Geometry: see drawing. Coordinates: mm, zero at the bounding-box minimum. A direction names the side the tool comes from. Round coordinates to 2 decimals unless told otherwise and drop trailing zeros. Order: outer loops, then holes, each group sorted by start corner. A loop starts at its lowest first (then second) coordinate and runs counter-clockwise, first axis right, second up. Notation, with made-up numbers: (55.5, 47.25) -> (105.5, 47.25) arc R24 ccw to (105.5, 61.25) -> close; hole circle Ø5 at (-38, 27.5). An arc over 180 degrees is marked (long way). Answer as CSV lines item,"result". Start each with the question number.
(1) Contact query for flat-ended pins moving along their axis: P1, Ø5, axis at x = 5, z = 6, coming from the -Y side; P2, Ø3.5, axis at y = 6, z = 4, coming from the +X side; P3, Ø2.5, axis at y = 6, z = 5, coming from the -X side. Output: stop coordinate, or through.
(2) Section query D-D (x = 28.5). Output: boundary loops of the cut face in (y, z).
(3) Section query A-A (y = 4.75). Output: boundary loops of the cut face in (x, z).
(4) Section query C-C (y = 1.5). Output: boundary loops of the cut face in (x, z), plus the area to 3 significant figures.
(5) Pull-direction query (Z, two-part tool) for the marked faces 1, 2, 3 and 4; classes: +Z half, -Z half, draft (parallel to the pull), parting line (faces both ways), or undercut.
(6) Section query B-B (z = 3.5). Output: boundary loops of the cut face in (x, y).
(7) Line query: line 1 along X through (y, z) = (4.25, 5); line 2 along X through (y, z) = (0.4, 5); line 3 along X through (y, z) = (6.5, 9). Output: solid intervals per line, ascending. Write a range as from..to.
(8) Set-up query: the marked faces 5, 6 and 7. Return all of +Z, -Z, +X, -X, +Y, -Y with unobstructed straight access to the full face (end or side cutting, diameter ignored); none if empty.
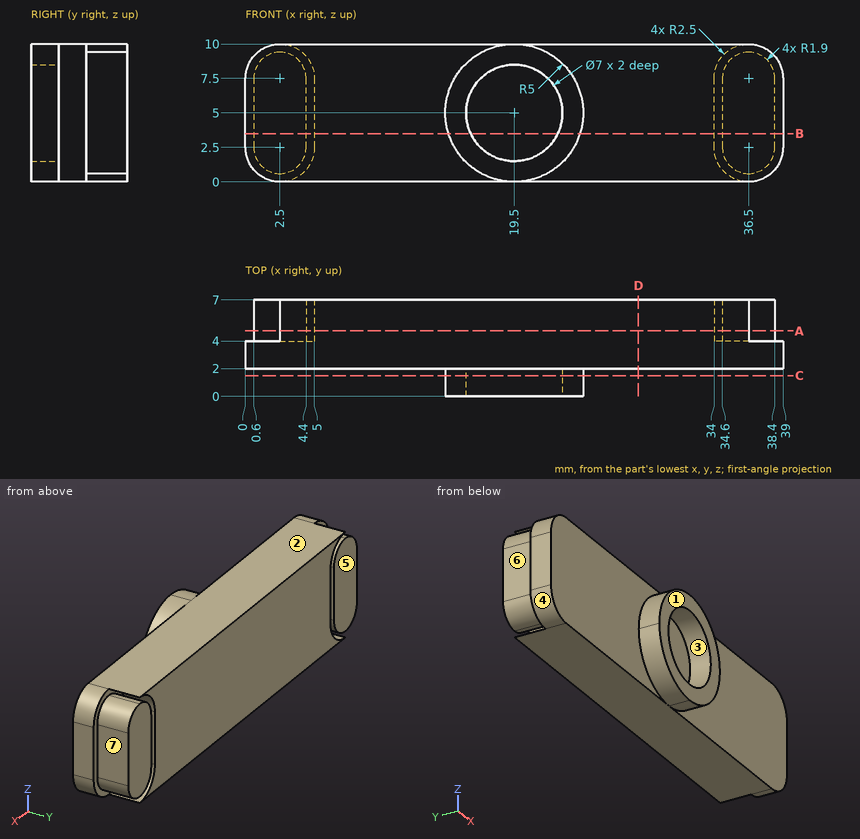
Answer block:
1,P1,"y = 2"
1,P2,"x = 38.4"
1,P3,"x = 0.6"
2,outline,"(2, 0) -> (7, 0) -> (7, 10) -> (2, 10) -> close"
3,outline,"(0.6, 2.5) arc R1.9 ccw to (4.4, 2.5) -> (4.4, 7.5) arc R1.9 ccw to (0.6, 7.5) -> close; (2.5, 0) -> (36.5, 0) arc R2.5 cw to (34, 2.5) -> (34, 7.5) arc R2.5 cw to (36.5, 10) -> (2.5, 10) arc R2.5 cw to (5, 7.5) -> (5, 2.5) arc R2.5 cw to start; (34.6, 2.5) arc R1.9 ccw to (38.4, 2.5) -> (38.4, 7.5) arc R1.9 ccw to (34.6, 7.5) -> close"
4,outline,"circle Ø10 at (19.5, 5); hole circle Ø7 at (19.5, 5)"
4,area,"40.1 mm2"
5,face 1,"draft"
5,face 2,"+Z half"
5,face 3,"undercut"
5,face 4,"-Z half"
6,outline,"(0, 2) -> (14.73, 2) -> (14.73, 0) -> (16.34, 0) -> (16.34, 2) -> (22.66, 2) -> (22.66, 0) -> (24.27, 0) -> (24.27, 2) -> (39, 2) -> (39, 4) -> (38.4, 4) -> (38.4, 7) -> (34.6, 7) -> (34.6, 4) -> (34, 4) -> (34, 7) -> (5, 7) -> (5, 4) -> (4.4, 4) -> (4.4, 7) -> (0.6, 7) -> (0.6, 4) -> (0, 4) -> close"
7,line 1,"0.6..4.4, 5..34, 34.6..38.4"
7,line 2,"14.5..16, 23..24.5"
7,line 3,"1.33..3.67, 4.5..34.5, 35.33..37.67"
8,face 5,"+Z, -Z, +X, -X, +Y"
8,face 6,"+Z, -Z, -X, +Y"
8,face 7,"+Z, -Z, +X, +Y"
